```python
from build123d import *

# Parameters (mm, degrees)
F1_DEPTH = 10
F2_R     = 2
F3_R     = 9.75
F4_DEPTH = 3
F5_R     = 0.5
F6_R     = 1


with BuildPart() as f1:
    # F0 (on Front) → F1 (new body)
    with BuildSketch(Plane.XZ):
        with BuildLine():
            Line((0, 23), (0, 0))
            Line((0, 0), (32.603637, 0))
            ThreePointArc((32.603637, 0), (35.903773, 2.769143), (33.749762, 6.5))
            ThreePointArc((33.749762, 6.5), (37.049899, 9.269143), (34.895887, 13))
            ThreePointArc((34.895887, 13), (38.196024, 15.769143), (36.042013, 19.5))
            ThreePointArc((36.042013, 19.5), (39.342149, 22.269143), (37.188138, 26))
            Line((37.188138, 26), (26, 26))
            ThreePointArc((26, 26), (23.87868, 26.87868), (23, 29))
            Line((23, 29), (23, 38))
            ThreePointArc((23, 38), (19, 39.527864), (15, 38))
            Line((15, 38), (15, 31.660254))
            Line((15, 31.660254), (11.443376, 25.5))
            ThreePointArc((11.443376, 25.5), (9.613249, 23.669873), (7.113249, 23))
            Line((7.113249, 23), (0, 23))
        make_face()
    extrude(amount=F1_DEPTH)

    # F2
    f2_edges = [f1.edges().sort_by_distance(p)[0] for p in [
        (37.188138, -5, 26),
        (23, -5, 38),
        (15, -5, 38),
        (15, -5, 31.660254),
        (0, -5, 23),
        (0, -5, 0),
    ]]
    fillet(f2_edges, radius=F2_R)

    # F3 (on face) → F4 (cut)
    with BuildSketch(Plane(origin=(0, 0, 0), x_dir=(-1, 0, 0), z_dir=(0, 1, 0))):
        with Locations((-18, 13)):
            Circle(F3_R)
    extrude(amount=-F4_DEPTH, mode=Mode.SUBTRACT)

    # F5
    f5_edges = [f1.edges().sort_by_distance(p)[0] for p in [
        (33.749762, -5, 6.5),
        (34.895887, -5, 13),
        (36.042013, -5, 19.5),
    ]]
    fillet(f5_edges, radius=F5_R)

    # F6
    f6_edges = [f1.edges().sort_by_distance(p)[0] for p in [
        (35.742216, -10, 2.176809),
        (34.638998, -10, 6.343204),
        (17.301818, -10, 0),
        (37.049899, -10, 9.269143),
        (0.585786, -10, 0.585786),
        (35.785124, -10, 12.843204),
        (0, -10, 11.5),
        (38.196024, -10, 15.769143),
        (0.585786, -10, 22.414214),
        (36.931249, -10, 19.343204),
        (4.556624, -10, 23),
        (39.378411, -10, 22.538066),
        (9.613249, -10, 23.669873),
        (37.299769, -10, 25.923755),
        (13.087713, -10, 28.348076),
        (31.376405, -10, 26),
        (14.931852, -10, 31.678514),
        (23.87868, -10, 26.87868),
        (15, -10, 34.594059),
        (23, -10, 32.995983),
        (15.267949, -10, 37.991966),
        (22.732051, -10, 37.991966),
        (19, -10, 39.527864),
    ]]
    fillet(f6_edges, radius=F6_R)


solid = f1.part
```
Geometry: final body of the model. Coordinates: model frame, mm. A direction names the side the tool comes from. Round coordinates to 2 decimals unless told otherwise and drop trailing zeros. Loops run counter-clockwise (first coordinate to the right, second up) from the corner with the lowest first, then second, coordinate; pieces in that order, holes last. Notation, with made-up numbers: (-20.5, -15.5) -> (19.5, -15.5) arc R23 ccw to (19.5, 7.5) -> close; hole circle Ø5 at (83.5, 66). An arc over 180 degrees is marked (long way). Use one line per item in the form item = value.
Item 1: Cut plane A-A on z = 36. Output: boundary loops of the cut face in (x, y), then the cut area to 3 significant figures.
Evaluation:
outline = (15, -9) arc R1 ccw to (16, -10) -> (22, -10) arc R1 ccw to (23, -9) -> (23, 0) -> (15, 0) -> close
area = 79.6 mm2
Item 2: Access query for faces 4 (the flat face through (18, -3, 13)), 5 (the cylindrical face through (22.715, -9.699, 33.052)), 6 (the flat face through (23, -4, 33)), 7 (the cylindrical face through (15.285, -9.699, 34.56)). Directions: +Z, -Z, +X, -X, +Y, -Y. A direction counts if a zero-diameter tool reaches every point of the face in a straight line with its end or side. Return the directions, or none.
Evaluation:
face_4 = +Y
face_5 = +Z, +X, -Y
face_6 = +Z, +X, +Y, -Y
face_7 = +Z, -X, -Y
Item 3: Cut plane B-B on x = 5. Output: boundary loops of the cut face in (y, z).
Evaluation:
outline = (-10, 1) arc R1 ccw to (-9, 0) -> (0, 0) -> (0, 23) -> (-9, 23) arc R1 ccw to (-10, 22) -> close
Item 4: Contact query for flat-ended pins moving along their axis: pin 1 Ø2.5 at (y, z) = (-6, 31.5) entering from +X; pin 2 Ø1 at (y, z) = (-4, 23) entering from -X; pin 3 Ø10 at (x, z) = (19, 13.5) entering from +Y. Output: stop coordinate, or through.
Evaluation:
pin_1 = 23
pin_2 = 0.68
pin_3 = -3
Item 5: Material intervals for probe 1 along X at (y, z) = (-1, 35.5); probe 2 along Y at (x, z) = (18.5, 6); probe 3 along Z at (x, y) = (18, -1.1), sorted ascending.
Evaluation:
probe_1 = 15 to 23
probe_2 = -10 to -3
probe_3 = 0 to 3.25, 22.75 to 39.44
Item 6: Draft query along Z for faces 1 (the flat face through (19, -10, 16)), 2 (the cylindrical face through (9.645, -4.437, 23.688)), 3 (the cylindrical face through (13.5, -1.48, 4.35)). Return one class per face: released by +Z, released by -Z, zero draft, split by the parting line, or undercut.
Evaluation:
face_1 = zero draft
face_2 = released by +Z
face_3 = undercut
